Check sheet for the modelled part. Datum: model origin and axes. Units: mm. Face numbers are marked on the shaded views. Coordinates: 2 decimals unless noted, no trailing zeros. Loops run counter-clockwise (first coordinate to the right, second up) from the corner with the lowest first, then second, coordinate; pieces in that order, holes last.
```python
from build123d import *

# Parameters (mm, degrees)
SKETCH_W        = 180
SKETCH_H        = 180
SKETCH_W_2      = 163.5
SKETCH_H_2      = 98
PAD_DEPTH       = 2
SKETCH003_W     = 172
SKETCH003_H     = 111.5
POCKET001_DEPTH = 1
SKETCH002_W     = 22
SKETCH002_H     = 22
SKETCH002_W_2   = 15
SKETCH002_H_2   = 15
POCKET_DEPTH    = 1
SKETCH001_R     = 2.625
PAD001_DEPTH    = 5


with BuildPart() as part:
    # Sketch (on DatumPlane) → Pad (new body)
    with BuildSketch(Plane.XY.offset(-2)):
        Rectangle(SKETCH_W, SKETCH_H)
        Rectangle(SKETCH_W_2, SKETCH_H_2, mode=Mode.SUBTRACT)
    extrude(amount=PAD_DEPTH)

    # Sketch003 (on DatumPlane) → Pocket001 (cut)
    with BuildSketch(Plane.XY):
        with Locations((0, -3.75)):
            Rectangle(SKETCH003_W, SKETCH003_H)
    extrude(amount=-POCKET001_DEPTH, mode=Mode.SUBTRACT)

    # Sketch002 (on DatumPlane) → Pocket (cut)
    with BuildSketch(Plane.XY):
        with Locations((0, 70)):
            Rectangle(SKETCH002_W, SKETCH002_H)
        with Locations((0, -65)):
            Rectangle(SKETCH002_W_2, SKETCH002_H_2)
    extrude(amount=-POCKET_DEPTH, mode=Mode.SUBTRACT)

    # Sketch001 (on DatumPlane) → Pad001 (join)
    with BuildSketch(Plane.XY):
        with Locations((75, 75)):
            Circle(SKETCH001_R)
        with Locations((-75, 75)):
            Circle(SKETCH001_R)
        with Locations((-75, -75)):
            Circle(SKETCH001_R)
        with Locations((75, -75)):
            Circle(SKETCH001_R)
    extrude(amount=PAD001_DEPTH)


solid = part.part
```
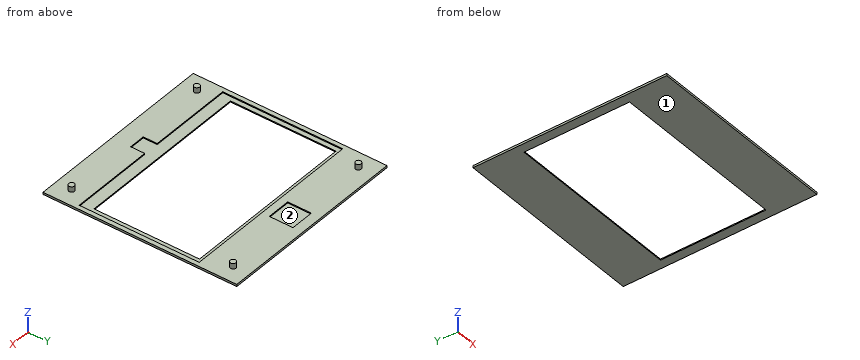
1) Mould release check, pull along X, two halves, no side actions. Record for the marked faces 1 and 2: +X half, -X half, draft (parallel to the pull), parting line (faces both ways), or undercut.
Answer sheet:
face 1: draft
face 2: undercut
2) Section check B-B on x = -75. Enter the section's corners in (y, z) (3 decimals), plus the area to 3 significant figures.
Answer sheet:
outline: (-90, -2) - (-49, -2) - (-49, -1) - (-59.5, -1) - (-59.5, 0) - (-72.375, 0) - (-72.375, 5) - (-77.625, 5) - (-77.625, 0) - (-90, 0) - close; (49, -2) - (90, -2) - (90, 0) - (77.625, 0) - (77.625, 5) - (72.375, 5) - (72.375, 0) - (52, 0) - (52, -1) - (49, -1) - close
area: 203 mm2
3) Section check A-A on y = 1. Enter the section's corners in (x, z).
Answer sheet:
outline: (-90, -2) - (-81.75, -2) - (-81.75, -1) - (-86, -1) - (-86, 0) - (-90, 0) - close; (81.75, -2) - (90, -2) - (90, 0) - (86, 0) - (86, -1) - (81.75, -1) - close
4) Section check D-D on x = 36.5. Enter the section's corners in (y, z).
Answer sheet:
outline: (-90, -2) - (-49, -2) - (-49, -1) - (-59.5, -1) - (-59.5, 0) - (-90, 0) - close; (49, -2) - (90, -2) - (90, 0) - (52, 0) - (52, -1) - (49, -1) - close
5) Scan lines: line 1 (X direction, y = 0, z = -0.5); line 2 (Y direction, x = 33.5, z = -0.5); line 3 (Z direction, x = 57.5, y = -54). Record each from-to range of solid material in increasing order.
Answer sheet:
line 1: x = -90 to -86, 86 to 90
line 2: y = -90 to -59.5, 52 to 90
line 3: z = -2 to -1
6) Section check C-C on y = 75. Enter the section's corners in (x, z) (3 decimals), plus the area to 4 significant figures.
Answer sheet:
outline: (-90, -2) - (90, -2) - (90, 0) - (77.625, 0) - (77.625, 5) - (72.375, 5) - (72.375, 0) - (11, 0) - (11, -1) - (-11, -1) - (-11, 0) - (-72.375, 0) - (-72.375, 5) - (-77.625, 5) - (-77.625, 0) - (-90, 0) - close
area: 390.5 mm2
